CAD build for the part. Positions are in the model's coordinates, mm. Face numbers are marked on the shaded views. A direction names the side the tool comes from. Give positions to 0.01 mm unless a question says otherwise; leave off trailing zeros. Loops run counter-clockwise (first coordinate to the right, second up) from the corner with the lowest first, then second, coordinate; pieces in that order, holes last. Notation, with made-up numbers: M -21,-33.5 L 16,-33.5 A27 cw 16,-0.5 Z; hole C 81.5,11.25 d9. An arc over 180 degrees is marked long. Answer as CSV lines item,"result".
from build123d import *

# Parameters (mm, degrees)
F0_W     = 63.6
F0_H     = 19.2
F1_DEPTH = 15.85
F2_R     = 4.7
F3_DEPTH = 4.9
F4_T     = -2.5
F5_R     = 6.8
F6_DEPTH = 16.5
F7_T     = -1


with BuildPart() as f1:
    # F0 (on Front) → F1 (new body, symmetric)
    with BuildSketch(Plane.XZ):
        with Locations((0, -9.6)):
            Rectangle(F0_W, F0_H)
    extrude(amount=F1_DEPTH, both=True)

    # F2 (on Top) → F3 (join)
    with BuildSketch(Plane.XY):
        with Locations((-24.2, 7.491081953)):
            Circle(F2_R)
        with Locations((-7.8, 7.491081953)):
            Circle(F2_R)
        with Locations((8.6, 7.491081953)):
            Circle(F2_R)
        with Locations((25, 7.491081953)):
            Circle(F2_R)
        with Locations((25, -7.491081953)):
            Circle(F2_R)
        with Locations((8.6, -7.491081953)):
            Circle(F2_R)
        with Locations((-7.8, -7.491081953)):
            Circle(F2_R)
        with Locations((-24.2, -7.491081953)):
            Circle(F2_R)
    extrude(amount=F3_DEPTH)

    # F4
    f4_openings = [f1.faces().sort_by_distance(p)[0] for p in [
        (0, 0, -19.2),
    ]]
    offset(amount=F4_T, openings=f4_openings, kind=Kind.INTERSECTION)

    # F5 (on Top) → F6 (join)
    with BuildSketch(Plane.XY):
        with BuildLine():
            ThreePointArc((9.7, 0), (16.5, -6.8), (23.3, 0))
            ThreePointArc((23.3, 0), (16.5, 6.8), (9.7, 0))
        make_face()
        with Locations((-16.3, 0)):
            Circle(F5_R)
        with BuildLine():
            ThreePointArc((0, -6.7992646661), (4.8728398255, -4.8435524153), (6.9, 0))
            ThreePointArc((6.9, 0), (4.9083261121, 4.8083261121), (0.1, 6.8))
            ThreePointArc((0.1, 6.8), (-4.7083261121, 4.8083261121), (-6.7, 0))
            ThreePointArc((-6.7, 0), (-4.7435524153, -4.7728398255), (0, -6.7992646661))
        make_face()
    extrude(amount=-F6_DEPTH)

    # F7
    f7_openings = [f1.faces().sort_by_distance(p)[0] for p in [
        (16.5, 0, -16.5),
        (0.1, 0, -16.5),
        (-16.3, 0, -16.5),
        (-24.2, -7.491082, 4.9),
        (-24.2, 7.491082, 4.9),
        (-7.8, 7.491082, 4.9),
        (-7.8, -7.491082, 4.9),
        (8.6, -7.491082, 4.9),
        (8.6, 7.491082, 4.9),
        (25, 7.491082, 4.9),
        (25, -7.491082, 4.9),
    ]]
    offset(amount=F7_T, openings=f7_openings, kind=Kind.INTERSECTION)


solid = f1.part
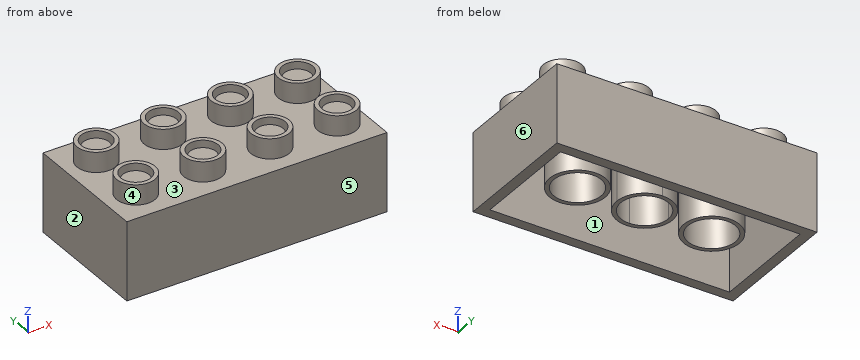
1) Flat gauge pins, fed straight in: pin 1 (5 mm diameter, centred on x = -24.5, y = 6.5, fed in from -Z); pin 2 (3 mm diameter, centred on x = -8.5, y = 7, fed in from +Z); pin 3 (4 mm diameter, centred on x = 18, y = -2.5, fed in from -Z). Where does each tip first touch, or does it go through?
Answer below:
pin 1,"stops at z = -2.5"
pin 2,"stops at z = 3.4"
pin 3,"stops at z = -1"
2) Mould opens along Y. For the marked faces 4, 5 and 6 say: +Y half, -Y half, draft (parallel to the pull), parting line (faces both ways), or undercut.
Answer below:
face 4,"undercut"
face 5,"-Y half"
face 6,"draft"
3) Band-saw the part on A-A on z = -15.5. Give the number of separate pieces and of enclosed holes in the cut face, and give its area (3 significant figures).
Answer below:
separate pieces,"5"
enclosed holes,"5"
area,"480 mm^2"
4) Band-saw the part on B-B on x = -16.3. Give the cut face in (y, z).
Answer below:
outline,"M -15.85,-19.2 L -13.35,-19.2 L -13.35,-2.5 L -6.8,-2.5 L -6.8,-16.5 L -5.8,-16.5 L -5.8,-1.5 L -14.35,-1.5 L -14.35,-18.2 L -14.85,-18.2 L -14.85,-1 L 14.85,-1 L 14.85,-18.2 L 14.35,-18.2 L 14.35,-1.5 L 5.8,-1.5 L 5.8,-16.5 L 6.8,-16.5 L 6.8,-2.5 L 13.35,-2.5 L 13.35,-19.2 L 15.85,-19.2 L 15.85,0 L -15.85,0 Z"
5) Drill centre lines: line 1 (X direction, y = 10.5, z = -4); line 2 (Y direction, x = -24, z = -8.25); line 3 (X direction, y = -13.5, z = -16.25). Where is each one in solid material? Low to high. Write a range as from..to.
Answer below:
line 1,"x = -31.8..-30.8, -30.3..-29.3, 29.3..30.3, 30.8..31.8"
line 2,"y = -15.85..-14.85, -14.35..-13.35, 13.35..14.35, 14.85..15.85"
line 3,"x = -31.8..-30.8, -30.3..30.3, 30.8..31.8"
6) Which spindle directions (+Z, -Z, +X, -X, +Y, -Y) get a long thin tool onto all of the face, cutting with end or side? Do the marked faces 1, 2 and 3. Say none if no direction does.
Answer below:
face 1,"-Z"
face 2,"+Z, -Z, -X, +Y, -Y"
face 3,"+Z"
